Autodesk Inventor part; units mm, degrees
ref_plane "YZ Plane" through (0, 0, 0) normal (1, 0, 0) x (0, 1, 0)
ref_plane "XZ Plane" through (0, 0, 0) normal (0, 1, 0) x (-1, 0, 0)
ref_plane "XY Plane" through (0, 0, 0) normal (0, 0, 1) x (1, 0, 0)
sketch "Esboço1" plane through (0, 0, 0) normal (0, 1, 0) x (-1, 0, 0)
  line L0 (0, 0) -> (80, 0)
  line L1 (80, 0) -> (80, -80)
  line L2 (80, -80) -> (0, -80)
  line L3 (0, -80) -> (0, 0)
  dimension "d0" = 80
  dimension "d1" = 80
extrude "Extrusão1" add sketch "Esboço1" along normal blind 6
sketch "Esboço2" plane through (0, 6, 0) normal (0, 1, 0) x (1, 0, 0)
  line L0 (-80, 0) -> (0, 0)
  line L1 (0, 0) -> (0, 80)
  point P0 (-16.4, 16.4)
  point P1 (-16.4, 63.6)
  point P2 (-63.6, 63.6)
  point P3 (-63.6, 16.4)
  dimension "d4" = 47.2
  dimension "d5" = 47.2
  dimension "d6" = 47.2
  dimension "d7" = 47.2
  dimension "d8" = 0
  dimension "d9" = 0
  dimension "d10" = 80
  dimension "d11" = 16.4
  dimension "d12" = 16.4
hole "Furo1" at (-16.4, 6, -16.4) at (-16.4, 6, -63.6) at (-63.6, 6, -63.6) at (-63.6, 6, -16.4) direction (0, -1, 0) diameter 5 depth 6
sketch "Esboço3" plane through (0, 6, 0) normal (0, 1, 0) x (1, 0, 0)
  line L0 (-80, 0) -> (0, 0)
  line L1 (-80, 80) -> (-80, 0)
  line L2 (0, 0) -> (0, 80)
  line L3 (0, 80) -> (-80, 80)
  point P0 (-8, 8)
  point P1 (-8, 72)
  point P2 (-72, 72)
  point P3 (-72, 8)
  dimension "d20" = 8
  dimension "d21" = 8
  dimension "d22" = 8
  dimension "d23" = 8
  dimension "d24" = 8
  dimension "d25" = 8
  dimension "d26" = 8
  dimension "d27" = 8
hole "Furo2" at (-8, 6, -8) at (-8, 6, -72) at (-72, 6, -72) at (-72, 6, -8) direction (0, -1, 0) diameter 5 depth 6
sketch "Esboço4" plane through (0, 6, 0) normal (0, 1, 0) x (1, 0, 0)
  line L0 (-80, 80) -> (-80, 0)
  line L1 (-80, 0) -> (0, 0)
  point P0 (-40, 40)
  dimension "d35" = 80
  dimension "d36" = 40
  dimension "d37" = 40
hole "Furo3" at (-40, 6, -40) direction (0, -1, 0) diameter 10 depth 6
equation "\"d18\" = Espessura"
equation "\"Raio_vergadura\" = Espessura"
equation "\"Largura_alívio_de_vergadura\" = Espessura"
equation "\"Profundidade_alívio_de_vergadura\" = 0.5 * Espessura"
equation "\"Tamanho_alívio_de_dobra\" = 4 * Espessura"
equation "\"Remanescente_mínimo\" = 2 * Espessura"
equation "\"Raiodetransição\" = Raio_vergadura"
equation "\"Tamanho_de_raio_de_Jacobi\" = Raio_vergadura"
equation "\"TamanhoFolga\" = Espessura"
properties part number "Suporte do motor" material "Steel"
Can you work these out from the model? Positions are in its coordinate system, mm. Give positions to 0.01 mm unless a question says otherwise; leave off trailing zeros. Loops run counter-clockwise (first coordinate to the right, second up) from the corner with the lowest first, then second, coordinate; pieces in that order, holes last. Notation, with made-up numbers: M 5.5,77 L 34.5,77 A25 ccw 34.5,90 Z; hole C 27,52.5 d8. An arc over 180 degrees is marked long. Use one line per item in the form item = value. Start each with the question number.
(1) I want a section at C-C, the plane z = -63.6. Write out the boundary of the cut face in (x, y).
(2) Please list where these lines run through material, in increasing order: line 1 (X direction, y = 3.1, z = -16.4); line 2 (Z direction, x = -8, y = 3.7).
(3) I want a section at A-A, the plane x = -8. Write out the boundary of the cut face in (y, z).
(4) Thinking about a two-plate mould opening in Z: for faces 1 (the cylindrical face through (-6.5, 3, -74)), 2 (the flat face through (-39, 3, 0)), 3 (the flat face through (-48, 0, -39)), which applies, released by +Z, released by -Z, zero draft, split by the parting line, or undercut?
(5) I want a section at D-D, the plane y = 2.85. State how many separate pieces and enclosed holes the cut face has, and give its area (3 significant figures).
(6) I want a section at B-B, the plane z = -40. Write out the boundary of the cut face in (x, y), and give its area (3 significant figures).
Worked out:
q1.outline = M -80,0 L -66.1,0 L -66.1,6 L -80,6 Z; M -61.1,0 L -18.9,0 L -18.9,6 L -61.1,6 Z; M -13.9,0 L 0,0 L 0,6 L -13.9,6 Z
q2.line_1 = -80 to -66.1, -61.1 to -18.9, -13.9 to 0
q2.line_2 = -80 to -74.5, -69.5 to -10.5, -5.5 to 0
q3.outline = M 0,-80 L 6,-80 L 6,-74.5 L 0,-74.5 Z; M 0,-69.5 L 6,-69.5 L 6,-10.5 L 0,-10.5 Z; M 0,-5.5 L 6,-5.5 L 6,0 L 0,0 Z
q4.face_1 = undercut
q4.face_2 = released by +Z
q4.face_3 = zero draft
q5.separate_pieces = 1
q5.enclosed_holes = 9
q5.area = 6,160 mm²
q6.outline = M -80,0 L -45,0 L -45,6 L -80,6 Z; M -35,0 L 0,0 L 0,6 L -35,6 Z
q6.area = 420 mm²
